Here's the drawing with two shaded views (mm, measured from the low corner). I have some questions. A direction names the side the tool comes from. Coordinates: 2 decimals unless noted, no trailing zeros. Write each loop counter-clockwise with the first axis right and the second up, starting at its lowest first coordinate (ties: lowest second). Pieces come first, ordered by that corner, then holes.
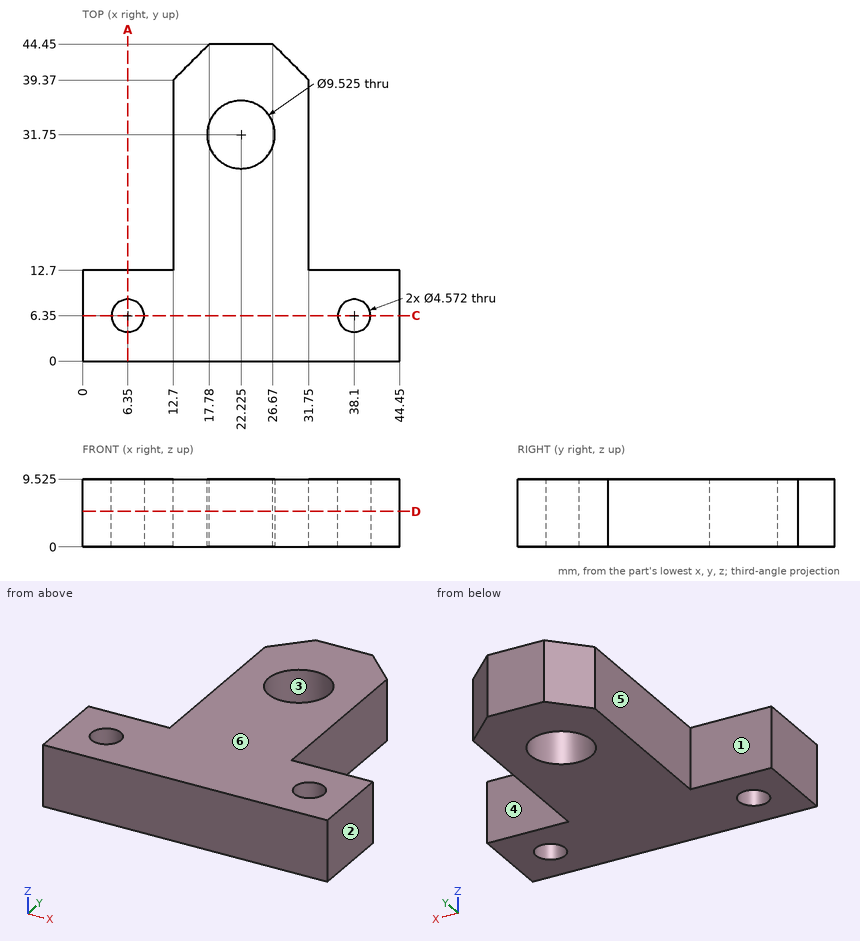
1. If I drill on L1, parallel to Y at x = 6.35, z = 3; L2, parallel to X at y = 7.5, z = 1; L3, parallel to Y at x = 9, z = 7.25, over which ranges is the centre line in solid material (lowest first)?
2. I'm going to push flat-ended pins straight in: P1, Ø2, axis at x = 14.5, z = 7, coming from the +Y side; P2, Ø5, axis at y = 25, z = 5, coming from the -X side; P3, Ø2.5, axis at x = 38.1, y = 6.35, coming from the -Z side; P4, Ø3, axis at x = 4, z = 5, coming from the +Y side. Where does each tip first touch, or does it pass through?
3. If we section it at D-D, the plane z = 5: Count the separate pieces of the cut face and the enclosed holes in it, plus the area to 3 significant figures.
4. If we section it at C-C, the plane y = 6.35: List the corners of the cut face in (x, z) for me (3 decimals), plus the area to 3 significant figures.
5. Which directions (+Z, -Z, +X, -X, +Y, -Y) give clear straight access to the entire face, cutting with the end or side of a thin tool? Please do the marked faces 4, 5 and 6.
6. If we section it at A-A, the plane x = 6.35: List the corners of the cut face in (y, z) for me (3 decimals).
7. We'd pull the mould along X, two halves only. Please class the marked faces 1, 2 and 3: released by +X, released by -X, zero draft, split by the parting line, or undercut.
Answers:
1. L1: y = 0 to 4.06, 8.64 to 12.7
1. L2: x = 0 to 4.37, 8.33 to 36.12, 40.08 to 44.45
1. L3: y = 0 to 12.7
2. P1: stops at y = 42.17
2. P2: stops at x = 12.7
2. P3: passes through
2. P4: stops at y = 12.7
3. separate pieces: 1
3. enclosed holes: 3
3. area: 1,040 mm2
4. outline: (0, 0) - (4.064, 0) - (4.064, 9.525) - (0, 9.525) - close; (8.636, 0) - (35.814, 0) - (35.814, 9.525) - (8.636, 9.525) - close; (40.386, 0) - (44.45, 0) - (44.45, 9.525) - (40.386, 9.525) - close
4. area: 336 mm2
5. face 4: +Z, -Z, +X, +Y
5. face 5: +Z, -Z, -X, +Y
5. face 6: +Z, +X, -X, +Y, -Y
6. outline: (0, 0) - (4.064, 0) - (4.064, 9.525) - (0, 9.525) - close; (8.636, 0) - (12.7, 0) - (12.7, 9.525) - (8.636, 9.525) - close
7. face 1: zero draft
7. face 2: released by +X
7. face 3: undercut
